Geometry: final body of the model. Coordinates: model frame, mm. Round coordinates to 2 decimals unless told otherwise and drop trailing zeros. Loops run counter-clockwise (first coordinate to the right, second up) from the corner with the lowest first, then second, coordinate; pieces in that order, holes last. Notation, with made-up numbers: M 56.5,60.5 L 102.5,60.5 A26 cw 102.5,83.5 Z; hole C 69,7 d2. An arc over 180 degrees is marked long. Return JSON: item names as keys, results as strings.
from build123d import *

# Parameters (mm, degrees)
SKETCH_1_W          = 65.5
SKETCH_1_H          = 65.5
EXTRUDE_1_DEPTH     = 5
FILLET_1_R          = 5
SKETCH_7_R          = 3.2
CUT_EXTRUDE_2_DEPTH = 5
CUT_EXTRUDE_START   = -15
SKETCH_3_R          = 3.2
CUT_EXTRUDE_3_DEPTH = 15
EXTRUDE_START       = -5
SKETCH_12_R         = 3.2
EXTRUDE_3_DEPTH     = 5


with BuildPart() as part:
    # 스케치1 → 보스-돌출1 (new body)
    with BuildSketch(Plane.XY):
        Rectangle(SKETCH_1_W, SKETCH_1_H)
    extrude(amount=EXTRUDE_1_DEPTH)

    # 필렛1
    fillet_1_edges = [part.edges().sort_by_distance(p)[0] for p in [
        (-32.75, -32.75, 2.5),
        (32.75, -32.75, 2.5),
        (32.75, 32.75, 2.5),
        (-32.75, 32.75, 2.5),
    ]]
    fillet(fillet_1_edges, radius=FILLET_1_R)

    # 스케치7 → 컷-돌출2 (cut)
    with BuildSketch(Plane(origin=(0, 0, 0), x_dir=(-1, 0, 0), z_dir=(0, 0, -1))):
        with Locations((-25, -25)):
            Circle(SKETCH_7_R)
        with Locations((-25, 25)):
            Circle(SKETCH_7_R)
    extrude(amount=-CUT_EXTRUDE_2_DEPTH, mode=Mode.SUBTRACT)

    # 스케치3 → 컷-돌출3 (cut)
    with BuildSketch(Plane.XY.offset(5).offset(CUT_EXTRUDE_START)):
        with Locations(Location((25, -25, 0), (0, 0, 180))):
            Circle(SKETCH_3_R)
        with Locations(Location((25, 25, 0), (0, 0, 180))):
            Circle(SKETCH_3_R)
        with Locations((25, 0)):
            Circle(SKETCH_3_R)
        with Locations((0, -25)):
            Circle(SKETCH_3_R)
        with Locations((0, 25)):
            Circle(SKETCH_3_R)
        Circle(SKETCH_3_R)
        with Locations((-25, -25)):
            Circle(SKETCH_3_R)
        with Locations((-25, 25)):
            Circle(SKETCH_3_R)
        with Locations((-25, 0)):
            Circle(SKETCH_3_R)
    extrude(amount=CUT_EXTRUDE_3_DEPTH, mode=Mode.SUBTRACT)

    # 스케치12 → 보스-돌출3 (add)
    with BuildSketch(Plane.XY.offset(5).offset(EXTRUDE_START)):
        with Locations((25, 0)):
            Circle(SKETCH_12_R)
        Circle(SKETCH_12_R)
        with Locations((0, -25)):
            Circle(SKETCH_12_R)
        with Locations((0, 25)):
            Circle(SKETCH_12_R)
        with Locations((-25, 0)):
            Circle(SKETCH_12_R)
    extrude(amount=EXTRUDE_3_DEPTH)


solid = part.part
Q1. Pin query (flat end, axial travel): pin 1 (6 mm diameter, centred on x = -25, y = 25, fed in from +Z). Return the tip coordinate at first contact, or that it passes through.
Determined:
{"pin 1": "passes through"}
Q2. Pull-direction query (Y, two-part tool) for faces 1 (the cylindrical face through (28.2, 25.1, 2.5)), 2 (the flat face through (0, 32.75, 2)), 3 (the flat face through (-32.75, 0, 2)); classes: pulls with the +Y half, pulls with the -Y half, needs draft (parallel to the pull), parting line crosses it, or undercut.
Determined:
{"face 1": "undercut", "face 2": "pulls with the +Y half", "face 3": "needs draft"}
Q3. Material intervals for L1, parallel to Y at x = 25, z = 2.3; L2, parallel to X at y = -29, z = 0.7; L3, parallel to X at y = 28.5, z = 3.7, sorted ascending.
Determined:
{"L1": "y = -32.75 to -28.2, -21.8 to 21.8, 28.2 to 32.75", "L2": "x = -32.59 to 32.59", "L3": "x = -32.69 to 32.69"}
Q4. Section query C-C (z = 4). Output: boundary loops of the cut face in (x, y).
Determined:
{"outline": "M -32.75,-27.75 A5 ccw -27.75,-32.75 L 27.75,-32.75 A5 ccw 32.75,-27.75 L 32.75,27.75 A5 ccw 27.75,32.75 L -27.75,32.75 A5 ccw -32.75,27.75 Z; hole C -25,-25 d6.4; hole C -25,25 d6.4; hole C 25,-25 d6.4; hole C 25,25 d6.4"}
Q5. Section query A-A (x = -25). Output: boundary loops of the cut face in (y, z), plus the area to 4 significant figures.
Determined:
{"outline": "M -32.75,0 L -28.2,0 L -28.2,5 L -32.75,5 Z; M -21.8,0 L 21.8,0 L 21.8,5 L -21.8,5 Z; M 28.2,0 L 32.75,0 L 32.75,5 L 28.2,5 Z", "area": "263.5 mm^2"}
